Geometry: final body of the model. Coordinates: model frame, mm. A direction names the side the tool comes from. Coordinates: 2 decimals unless noted, no trailing zeros. Order: outer loops, then holes, each group sorted by start corner. A loop starts at its lowest first (then second) coordinate and runs counter-clockwise, first axis right, second up. Notation, with made-up numbers: (14.25, 45) - (30.25, 45) arc R32 ccw to (30.25, 75) - close; hole circle Ø6 at (-9, -31.5). An arc over 180 degrees is marked (long way). Use a Markdown table: item, result. Add a question column.
```python
from build123d import *

# Parameters (mm, degrees)
BOSS_EXTRUDE1_DEPTH          = 0.635
F_97_0_0059_DIAMETER_HOLE1_D = 2.921
SKETCH5_W                    = 19.05
SKETCH5_H                    = 0.762
CUT_EXTRUDE1_DEPTH           = 0.635
FILLET4_R                    = 1.27
FILLET5_R                    = 1.27


with BuildPart() as part:
    # Sketch1 → Boss-Extrude1 (new, symmetric)
    with BuildSketch(Plane(origin=(0, 0, 0), x_dir=(1, 0, 0), z_dir=(0, 1, 0))):
        Polygon((-41.424046485, -10.283259465), (-41.424046485, -12.505759465), (-47.774046485, -12.505759465), (-47.774046485, -6.155759465), (-41.424046485, -6.155759465), (-41.424046485, -8.378259465), (-9.674046485, -8.378259465), (-9.674046485, -6.155759465), (-3.324046485, -6.155759465), (-3.324046485, -12.505759465), (-9.674046485, -12.505759465), (-9.674046485, -10.283259465), align=None)
    extrude(amount=BOSS_EXTRUDE1_DEPTH, both=True)

    # #97 (0.0059) Diameter Hole1 (through all)
    with Locations(Plane(origin=(0, 0.635, 0), x_dir=(-1, 0, 0), z_dir=(0, 1, 0))):
        with Locations((44.599046485, 9.330759465)):
            f_97_0_0059_diameter_hole1 = Hole(F_97_0_0059_DIAMETER_HOLE1_D / 2)

    # Mirror1: #97 (0.0059) Diameter Hole1 across plane
    add(f_97_0_0059_diameter_hole1.mirror(Plane(origin=(-25.549046485, 0, 0), x_dir=(0, 0, 1), z_dir=(1, 0, 0))), mode=Mode.SUBTRACT)

    # Sketch5 → Cut-Extrude1 (cut)
    with BuildSketch(Plane(origin=(0, 0.635, 0), x_dir=(1, 0, 0), z_dir=(0, 1, 0))):
        with Locations((-25.549046485, -9.902259465)):
            Rectangle(SKETCH5_W, SKETCH5_H)
    extrude(amount=-CUT_EXTRUDE1_DEPTH, mode=Mode.SUBTRACT)

    # Fillet4
    # the kernel refuses this fillet: 1.27 mm, written as the material it adds along each edge
    with BuildSketch(Plane(origin=(-35.074046485, 0.635, 9.521259465), x_dir=(0, 0, 1), z_dir=(0, -1, 0))) as fillet4_piece_1:
        with BuildLine():
            CenterArc((1.27, -1.163974227), FILLET4_R, 113.578178478, 66.421821522)
            Line((0, -1.163974227), (-0.0254, -1.163974227))
            Line((-0.0254, -1.163974227), (-0.0254, 0))
            Line((-0.0254, 0), (0, 0.0254))
            ThreePointArc((0, 0.0254), (0.381, 0.0254), (0.75184, 0.023279485))
            Line((0.75184, 0.023279485), (0.762, 0))
        make_face()
    extrude(amount=0.635)

    # Fillet5
    # the kernel refuses this fillet: 1.27 mm, written as the material it adds along each edge
    with BuildSketch(Plane(origin=(-16.024046485, 0.635, 9.521259465), x_dir=(-1, 0, 0), z_dir=(0, -1, 0))) as fillet5_piece_1:
        with BuildLine():
            CenterArc((1.163974227, -1.27), FILLET5_R, 90, 66.421821522)
            Line((0, -0.762), (-0.023279485, -0.75184))
            ThreePointArc((-0.023279485, -0.75184), (-0.0254, -0.381), (-0.0254, 0))
            Line((-0.0254, 0), (0, 0.0254))
            Line((0, 0.0254), (1.163974227, 0.0254))
            Line((1.163974227, 0.0254), (1.163974227, 0))
        make_face()
    extrude(amount=0.635)


solid = part.part
```
1) Line query: line 1 (X direction, y = -0.1, z = 10); line 2 (X direction, y = 0.3, z = 10.5); line 3 (X direction, y = 0.2, z = 6.75). Output: solid intervals per line, ascending. Write a range as from..to.
2) Draft query along X for faces 1 (the flat face through (-3.324, 0, 9)), 2 (the cylindrical face through (-5.423, -0.009, 10.318)), 3 (the flat face through (-7, 0, 6.156)), 4 (the flat face through (-47.774, 0, 9)). Return one class per face: released by +X, released by -X, zero draft, split by the parting line, or undercut.
3) Section query A-A (z = 11.25). Return the cut outline in (x, y) (3 decimals), and give its area (3 significant figures).
4) Section query B-B (y = 0.35). Return the cut outline in (x, z), and give its area (3 significant figures).
5) Access query for faces 5 (the flat face through (-9.674, 0, 7)), 6 (the flat face through (-9.674, 0, 11)), 7 (the flat face through (-45, 0, 6.156)). Directions: +Z, -Z, +X, -X, +Y, -Y. A direction counts if a zero-diameter tool reaches every point of the face in a straight line with its end or side. Return the directions, or none.
6) Section query C-C (x = -20.5). Return the cut outline in (y, z) (3 decimals), and give its area (3 significant figures).
7) Section query D-D (x = -37.5). Return the cut outline in (y, z) (3 decimals), and give its area (3 significant figures).
8) First-contact query: pin 1 (1.5 mm diameter, centred on x = -22, z = 7.5, fed in from -Y); pin 2 (0.5 mm diameter, centred on x = -22.5, y = 0.5, fed in from +Z); pin 3 (0.6 mm diameter, centred on x = -25.5, z = 10, fed in from +Y). Flat tips, straight axial feed; report the tip coordinate or a pass-through.
From the geometry:
| question | item | result |
|---|---|---|
| 1 | line 1 | x = -47.77..-45.9, -43.3..-7.8, -5.2..-3.32 |
| 1 | line 2 | x = -47.77..-45.47, -43.72..-41.42, -9.67..-7.37, -5.62..-3.32 |
| 1 | line 3 | x = -47.77..-41.42, -9.67..-3.32 |
| 2 | face 1 | released by +X |
| 2 | face 2 | undercut |
| 2 | face 3 | zero draft |
| 2 | face 4 | released by -X |
| 3 | outline | (-47.774, -0.635) - (-41.424, -0.635) - (-41.424, 0.635) - (-47.774, 0.635) - close; (-9.674, -0.635) - (-3.324, -0.635) - (-3.324, 0.635) - (-9.674, 0.635) - close |
| 3 | area | 16.1 mm^2 |
| 4 | outline | (-47.77, 6.16) - (-41.42, 6.16) - (-41.42, 8.38) - (-9.67, 8.38) - (-9.67, 6.16) - (-3.32, 6.16) - (-3.32, 12.51) - (-9.67, 12.51) - (-9.67, 10.28) - (-16.02, 10.28) arc R1.27 cw to (-17.19, 9.52) - (-33.91, 9.52) arc R1.27 cw to (-35.07, 10.28) - (-41.42, 10.28) - (-41.42, 12.51) - (-47.77, 12.51) - close; hole circle Ø2.92 at (-44.6, 9.33); hole circle Ø2.92 at (-6.5, 9.33) |
| 4 | area | 114 mm^2 |
| 5 | face 5 | -Z, +Y, -Y |
| 5 | face 6 | +Z, +Y, -Y |
| 5 | face 7 | -Z, +X, -X, +Y, -Y |
| 6 | outline | (-0.635, 8.378) - (0.635, 8.378) - (0.635, 9.521) - (0, 9.521) - (0, 10.283) - (-0.635, 10.283) - close |
| 6 | area | 1.94 mm^2 |
| 7 | outline | (-0.635, 8.378) - (0.635, 8.378) - (0.635, 10.283) - (-0.635, 10.283) - close |
| 7 | area | 2.42 mm^2 |
| 8 | pin 1 | passes through |
| 8 | pin 2 | stops at z = 9.52 |
| 8 | pin 3 | stops at y = 0 |
